Source: CAD feature listing. Evaluate the final solid. Frame: model axes, mm. Face numbers are marked on the shaded views. A direction names the side the tool comes from. Round coordinates to 2 decimals unless told otherwise and drop trailing zeros. Loops run counter-clockwise (first coordinate to the right, second up) from the corner with the lowest first, then second, coordinate; pieces in that order, holes last.
Item 1: Section query A-A on x = -33. Return loops of the section in (y, z), then the cut area to 3 significant figures.
Item 2: Ray query, L1, parallel to Z at x = 29, y = 29.5; L2, parallel to Z at x = 29, y = 36; L3, parallel to Y at x = -34, z = 52. Return the intervals inside material, ascending.
Item 3: Section query C-C on y = 43. Return loops of the section in (x, z), then the cut area to 3 significant figures.
Item 4: First-contact query: P1, Ø8.5, axis at x = 27, y = 30.5, coming from the +Z side; P2, Ø8, axis at y = 32.5, z = 42.5, coming from the +X side; P3, Ø1.6, axis at x = 2.5, y = 34.5, coming from the +Z side; P4, Ø12, axis at x = -33, y = 29.5, coming from the +Z side. Flat tips, straight axial feed; report the tip coordinate or a pass-through.
Item 5: Section query D-D on x = 0. Return loops of the section in (y, z), then the cut area to 3 significant figures.
Item 6: Pull-direction query (X, two-part tool) for the marked faces 1, 2 and 3; classes: released by +X, released by -X, zero draft, split by the parting line, or undercut.
Item 7: Section query B-B on z = 43.5. Return loops of the section in (x, y).
Item 8: Access query for the marked faces 4, 5 and 6. Directions: +Z, -Z, +X, -X, +Y, -Y. A direction counts if a zero-diameter tool reaches every point of the face in a straight line with its end or side. Return the directions, or none.
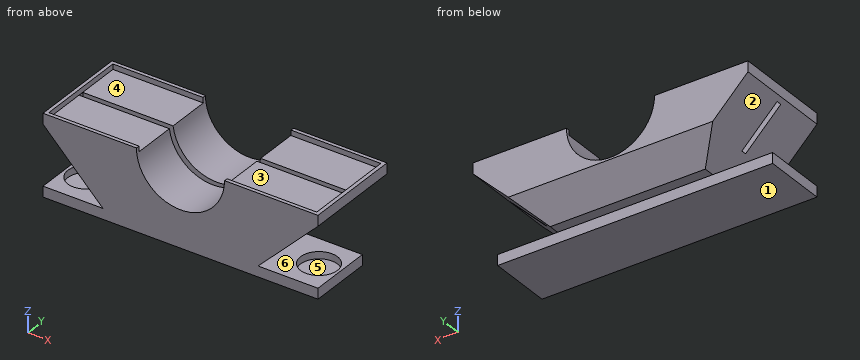
```python
from build123d import *

# Parameters (mm, degrees)
SKETCH071_W            = 78
SKETCH071_H            = 18
PAD022_DEPTH           = 3
SKETCH072_R            = 5.25
POCKET046_DEPTH        = 2
LINEARPATTERN002_COUNT = 2
LINEARPATTERN002_PITCH = 66
SKETCH073_W            = 78
SKETCH073_H            = 28
PAD023_DEPTH           = 20
POCKET050_DEPTH        = 28.001
SKETCH075_W            = 76
SKETCH075_H            = 26
POCKET047_DEPTH        = 1.5
SKETCH076_R            = 12.5
POCKET048_DEPTH        = 28.001
SKETCH077_W            = 76
SKETCH077_H            = 1.5
POCKET049_DEPTH        = 12.5
CHAMFER002_SIZE        = 7


with BuildPart() as part:
    # Sketch071 → Pad022 (new body)
    with BuildSketch(Plane.XY):
        with Locations((0, 29.5)):
            Rectangle(SKETCH071_W, SKETCH071_H)
    extrude(amount=PAD022_DEPTH)

    # Sketch072 (on Face6 of Pad022) → Pocket046 (cut)
    with BuildSketch(Plane.XY.offset(3)):
        with Locations((-33, 29.5)):
            Circle(SKETCH072_R)
    pocket046 = extrude(amount=-POCKET046_DEPTH, mode=Mode.SUBTRACT)

    # LinearPattern002: Pocket046 ×2
    with Locations(*[(i * LINEARPATTERN002_PITCH, 0, 0) for i in range(1, LINEARPATTERN002_COUNT)]):
        add(pocket046, mode=Mode.SUBTRACT)

    # Sketch073 (on Face5 of LinearPattern002) → Pad023 (join)
    with BuildSketch(Plane.XY.offset(3)):
        with Locations((0, 34.5)):
            Rectangle(SKETCH073_W, SKETCH073_H)
    extrude(amount=PAD023_DEPTH)

    # Sketch078 (on Face10 of Pad023) → Pocket050 (cut, through all)
    with BuildSketch(Plane.XZ.offset(-20.5)):
        Polygon((-39, 3), (-22, 3), (-39, 20), align=None)
        Polygon((39, 20), (39, 3), (22, 3), align=None)
    extrude(amount=-POCKET050_DEPTH, mode=Mode.SUBTRACT)

    # Sketch075 (on Face18 of Pocket050) → Pocket047 (cut)
    with BuildSketch(Plane.XY.offset(23)):
        with Locations((-0.049348, 34.5)):
            Rectangle(SKETCH075_W, SKETCH075_H)
    extrude(amount=-POCKET047_DEPTH, mode=Mode.SUBTRACT)

    # Sketch076 (on Face14 of Pocket047) → Pocket048 (cut, through all)
    with BuildSketch(Plane.XZ.offset(-20.5)):
        with Locations((0, 23)):
            Circle(SKETCH076_R)
    extrude(amount=-POCKET048_DEPTH, mode=Mode.SUBTRACT)

    # Sketch077 (on Face27 of Pocket048) → Pocket049 (cut)
    with BuildSketch(Plane.XY.offset(21.5)):
        with Locations((0, 34.5)):
            Rectangle(SKETCH077_W, SKETCH077_H)
    extrude(amount=-POCKET049_DEPTH, mode=Mode.SUBTRACT)

    # Chamfer002
    chamfer002_edges = [part.edges().sort_by_distance(p)[0] for p in [
        (0, 48.5, 3),
    ]]
    chamfer(chamfer002_edges, length=CHAMFER002_SIZE)


with BuildPart() as part_1:
    # Body006 placement: moved
    add(part.part.moved(Location((0, 0, 32))))


solid = part_1.part
```
Data:
1. outline: (20.5, 32) - (38.5, 32) - (38.5, 35) - (34.75, 35) - (34.75, 33) - (24.25, 33) - (24.25, 35) - (20.5, 35) - close; (20.5, 46) - (33.75, 46) - (33.75, 53.5) - (21.5, 53.5) - (21.5, 55) - (20.5, 55) - close; (35.25, 46) - (48.5, 46) - (48.5, 55) - (47.5, 55) - (47.5, 53.5) - (35.25, 53.5) - close
1. area: 235 mm2
2. L1: z = 32 to 33, 42 to 53.5
2. L2: z = 32 to 35, 42 to 53.5
2. L3: y = 20.5 to 33.75, 35.25 to 48.5
3. outline: (-39, 52) - (-23.5, 36.5) - (23.5, 36.5) - (39, 52) - (39, 55) - (37.95, 55) - (37.95, 53.5) - (12.41, 53.5) arc R12.5 cw to (-12.41, 53.5) - (-38.05, 53.5) - (-38.05, 55) - (-39, 55) - close
3. area: 881 mm2
4. P1: stops at z = 53.5
4. P2: stops at x = 33.5
4. P3: stops at z = 42.81
4. P4: stops at z = 55
5. outline: (20.5, 32) - (38.5, 32) - (38.5, 35) - (41.5, 35) - (48.5, 42) - (48.5, 42.5) - (35.25, 42.5) - (35.25, 41) - (33.75, 41) - (33.75, 42.5) - (20.5, 42.5) - close
5. area: 237 mm2
6. face 1: zero draft
6. face 2: released by -X
6. face 3: undercut
7. outline: (-30.5, 20.5) - (-4.9, 20.5) - (-4.9, 33.75) - (-30.5, 33.75) - close; (-30.5, 35.25) - (-4.9, 35.25) - (-4.9, 48.5) - (-30.5, 48.5) - close; (4.9, 20.5) - (30.5, 20.5) - (30.5, 33.75) - (4.9, 33.75) - close; (4.9, 35.25) - (30.5, 35.25) - (30.5, 48.5) - (4.9, 48.5) - close
8. face 4: +Z
8. face 5: none
8. face 6: +X, +Y, -Y
